Geometry: final body of the model. Coordinates: model frame, mm. Round coordinates to 2 decimals unless told otherwise and drop trailing zeros. Loops run counter-clockwise (first coordinate to the right, second up) from the corner with the lowest first, then second, coordinate; pieces in that order, holes last. Notation, with made-up numbers: M 83.25,64.5 L 110.25,64.5 A19 cw 110.25,99.5 Z; hole C 40,35.5 d3. An arc over 180 degrees is marked long. Return JSON: item names as keys, results as strings.
from build123d import *

# Parameters (mm, degrees)
SKETCH2_R           = 46.99
SKETCH2_R_2         = 1.5875
SKETCH2_R_3         = 22.240762899
BOSS_EXTRUDE1_DEPTH = 3.175


with BuildPart() as part:
    # Sketch2 → Boss-Extrude1 (new body)
    with BuildSketch(Plane.XY):
        Circle(SKETCH2_R)
        with Locations((0, -30.69717)):
            Circle(SKETCH2_R_2, mode=Mode.SUBTRACT)
        with Locations((0, 30.69717)):
            Circle(SKETCH2_R_2, mode=Mode.SUBTRACT)
        with Locations((30.69717, 0)):
            Circle(SKETCH2_R_2, mode=Mode.SUBTRACT)
        with Locations((-30.69717, 0)):
            Circle(SKETCH2_R_2, mode=Mode.SUBTRACT)
        Circle(SKETCH2_R_3, mode=Mode.SUBTRACT)
        Polygon((-19.05, -35.45967), (-15.875, -35.45967), (-15.875, -25.93467), (-19.05, -25.93467), (-19.05, -32.28467), align=None, mode=Mode.SUBTRACT)
        Polygon((-19.05, 32.28467), (-19.05, 35.45967), (-15.875, 35.45967), (-15.875, 25.93467), (-19.05, 25.93467), align=None, mode=Mode.SUBTRACT)
        Polygon((19.05, 35.45967), (15.875, 35.45967), (15.875, 25.93467), (19.05, 25.93467), (19.05, 32.28467), align=None, mode=Mode.SUBTRACT)
        Polygon((19.05, -32.28467), (19.05, -25.93467), (15.875, -25.93467), (15.875, -35.45967), (19.05, -35.45967), align=None, mode=Mode.SUBTRACT)
        Polygon((-35.45967, -19.05), (-35.45967, -15.875), (-25.93467, -15.875), (-25.93467, -19.05), (-32.28467, -19.05), align=None, mode=Mode.SUBTRACT)
        Polygon((-32.28467, 19.05), (-35.45967, 19.05), (-35.45967, 15.875), (-25.93467, 15.875), (-25.93467, 19.05), align=None, mode=Mode.SUBTRACT)
        Polygon((35.45967, 19.05), (35.45967, 15.875), (25.93467, 15.875), (25.93467, 19.05), (32.28467, 19.05), align=None, mode=Mode.SUBTRACT)
        Polygon((32.28467, -19.05), (35.45967, -19.05), (35.45967, -15.875), (25.93467, -15.875), (25.93467, -19.05), align=None, mode=Mode.SUBTRACT)
    extrude(amount=BOSS_EXTRUDE1_DEPTH)


solid = part.part
Q1. Section query A-A (y = 0). Output: boundary loops of the cut face in (x, z) (3 decimals).
Determined:
{"outline": "M -46.99,0 L -32.285,0 L -32.285,3.175 L -46.99,3.175 Z; M -29.11,0 L -22.241,0 L -22.241,3.175 L -29.11,3.175 Z; M 22.241,0 L 29.11,0 L 29.11,3.175 L 22.241,3.175 Z; M 32.285,0 L 46.99,0 L 46.99,3.175 L 32.285,3.175 Z"}
Q2. Section query C-C (y = 14). Output: boundary loops of the cut face in (x, z) (3 decimals).
Determined:
{"outline": "M -44.856,0 L -17.282,0 L -17.282,3.175 L -44.856,3.175 Z; M 17.282,0 L 44.856,0 L 44.856,3.175 L 17.282,3.175 Z"}
Q3. Pull-direction query (X, two-part tool) for faces 1 (the flat face through (-15.875, -31, 2)), 2 (the flat face through (9.8, -20.2, 0)); classes: pulls with the +X half, pulls with the -X half, needs draft (parallel to the pull), parting line crosses it, or undercut.
Determined:
{"face 1": "undercut", "face 2": "needs draft"}
Q4. Material intervals for L1, parallel to X at y = -28, z = 0.65 (3 decimals); L2, parallel to X at y = -32.5, z = 0.35 (3 decimals); L3, parallel to Y at x = -16.5, z = 1.95, sorted ascending.
Determined:
{"L1": "x = -37.737 to -19.05, -15.875 to 15.875, 19.05 to 37.737", "L2": "x = -33.938 to -19.05, -15.875 to 15.875, 19.05 to 33.938", "L3": "y = -44 to -35.46, -25.93 to -14.91, 14.91 to 25.93, 35.46 to 44"}
Q5. Section query D-D (y = -28). Output: boundary loops of the cut face in (x, z) (3 decimals).
Determined:
{"outline": "M -37.737,0 L -19.05,0 L -19.05,3.175 L -37.737,3.175 Z; M -15.875,0 L 15.875,0 L 15.875,3.175 L -15.875,3.175 Z; M 19.05,0 L 37.737,0 L 37.737,3.175 L 19.05,3.175 Z"}
Q6. Pin query (flat end, axial travel): pin 1 (3 mm diameter, centred on x = 0, y = 30.7, fed in from -Z); pin 2 (1.6 mm diameter, centred on y = -17, z = 2, fed in from +X); pin 3 (1 mm diameter, centred on y = 16.5, z = 2.5, fed in from -X); pin 4 (1 mm diameter, centred on y = 17.5, z = 1.5, fed in from +X). Return the tip coordinate at first contact, or that it passes through.
Determined:
{"pin 1": "passes through", "pin 2": "stops at x = 44.11", "pin 3": "stops at x = -44.18", "pin 4": "stops at x = 43.81"}
